Part model, mm, in its own coordinate system. Face numbers are marked on the shaded views. A direction names the side the tool comes from. Give positions to 0.01 mm unless a question says otherwise; leave off trailing zeros. One line per item, written item: value.
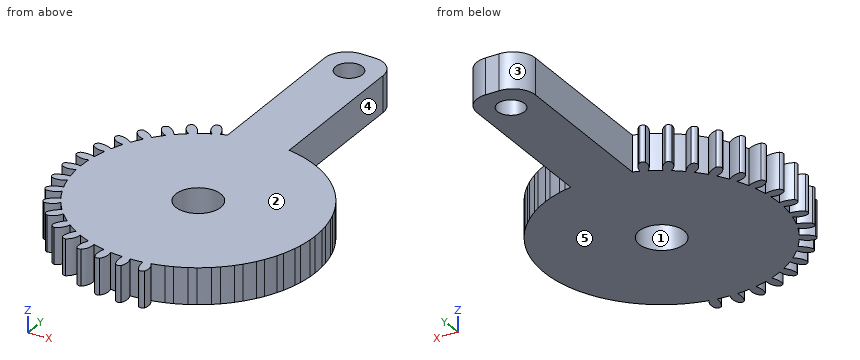
```python
from build123d import *

# Parameters (mm, degrees)
SKETCH1_R           = 13
BOSS_EXTRUDE1_DEPTH = 4
BOSS_EXTRUDE2_DEPTH = 4
CIRPATTERN1_COUNT   = 37
CUT_EXTRUDE1_START  = -6
CUT_EXTRUDE1_DEPTH  = 6
SKETCH5_W           = 6.5
SKETCH5_H           = 20
BOSS_EXTRUDE3_DEPTH = 4
FILLET1_R           = 2.5
SKETCH6_R           = 2.5
CUT_EXTRUDE2_DEPTH  = 36.685455193
SKETCH7_R           = 1.5
CUT_EXTRUDE3_DEPTH  = 36.685455193


with BuildPart() as part:
    # Sketch1 → Boss-Extrude1 (new body)
    with BuildSketch(Plane.XY):
        Circle(SKETCH1_R)
    extrude(amount=BOSS_EXTRUDE1_DEPTH)

    # Sketch2 → Boss-Extrude2 (add)
    with BuildSketch(Plane.XY.offset(4)):
        with BuildLine():
            Line((-1.442756516, 12.919692475), (-0.673396871, 12.982547387))
            ThreePointArc((-0.673396871, 12.982547387), (-0.676161598, 13.791154594), (-0.946073249, 14.553388784))
            ThreePointArc((-0.946073249, 14.553388784), (-1.263795502, 14.68499365), (-1.581517754, 14.553388784))
            ThreePointArc((-1.581517754, 14.553388784), (-1.735779337, 13.717545135), (-1.442756516, 12.919692475))
        make_face()
    boss_extrude2 = extrude(amount=-BOSS_EXTRUDE2_DEPTH)

    # CirPattern1: Boss-Extrude2 ×37 about axis
    cirpattern1_axis = Axis((-0.003550518, 0.04085181, 0), (0, 0, 1))
    for i in range(1, CIRPATTERN1_COUNT):
        add(boss_extrude2.rotate(cirpattern1_axis, i * 360 / CIRPATTERN1_COUNT))

    # Sketch3 → Cut-Extrude1 (cut)
    with BuildSketch(Plane.XY.offset(4).offset(CUT_EXTRUDE1_START)):
        with BuildLine():
            ThreePointArc((2.580226265, -12.741366976), (12.998773331, -0.178582984), (2.929279614, 12.665674911))
            ThreePointArc((2.929279614, 12.665674911), (2.706489738, 14.000196281), (3.492602617, 15.101381624))
            ThreePointArc((3.492602617, 15.101381624), (15.498537433, -0.212925866), (3.076423624, -15.191629856))
            ThreePointArc((3.076423624, -15.191629856), (3.335791003, -13.863732578), (2.580226265, -12.741366976))
        make_face()
    extrude(amount=CUT_EXTRUDE1_DEPTH, mode=Mode.SUBTRACT)

    # Sketch5 → Boss-Extrude3 (add)
    with BuildSketch(Plane.XY.offset(4)):
        with Locations((-1.029483868, 22.275423326)):
            Rectangle(SKETCH5_W, SKETCH5_H)
    extrude(amount=-BOSS_EXTRUDE3_DEPTH)

    # Fillet1
    fillet1_edges = [part.edges().sort_by_distance(p)[0] for p in [
        (2.220516132, 32.275423326, 2),
        (-4.279483868, 32.275423326, 2),
    ]]
    fillet(fillet1_edges, radius=FILLET1_R)

    # Sketch6 → Cut-Extrude2 (cut, through all)
    with BuildSketch(Plane.XY.offset(4)):
        Circle(SKETCH6_R)
    extrude(amount=-CUT_EXTRUDE2_DEPTH, mode=Mode.SUBTRACT)

    # Sketch7 → Cut-Extrude3 (cut, through all)
    with BuildSketch(Plane.XY.offset(4)):
        with Locations((-1.029483868, 28.906928641)):
            Circle(SKETCH7_R)
    extrude(amount=-CUT_EXTRUDE3_DEPTH, mode=Mode.SUBTRACT)


solid = part.part
```
1) Wall check: line 1 along Y through (x, z) = (-10.75, 0.65); line 2 along X through (y, z) = (18.5, 3.8); line 3 along Y through (x, z) = (0, 1.25). Give the ranges that are in metal, low to high. Write a range as [from, to].
Answer:
line 1: y = [-9.85, -8.78], [-7.31, 7.31], [7.49, 8.61]
line 2: x = [-4.28, 2.22]
line 3: y = [-14.66, -2.5], [2.5, 27.82], [30, 32.26]
2) Drop flat-ended pins along their axis: P1, Ø2, axis at y = -9.5, z = 2, coming from the -X side; P2, Ø4, axis at x = 0, y = 0, coming from the -Z side; P3, Ø1.2, axis at y = 18, z = 2, coming from the +X side; P4, Ø2, axis at y = 25, z = 1.5, coming from the -X side. Give the stop position or say it passes through.
Answer:
P1: stops at x = -11.12
P2: passes through
P3: stops at x = 2.22
P4: stops at x = -4.28
3) Two-plate mould, pull along Y, no slides. Class the marked faces 1, 2 and 3: pulls with the +Y half, pulls with the -Y half, needs draft (parallel to the pull), parting line crosses it, or undercut.
Answer:
face 1: undercut
face 2: needs draft
face 3: pulls with the +Y half
4) Which spindle directions (+Z, -Z, +X, -X, +Y, -Y) get a long thin tool onto all of the face, cutting with end or side? Do the marked faces 4 and 5. Say none if no direction does.
Answer:
face 4: +Z, -Z, +X, +Y
face 5: -Z, +X, -X, +Y, -Y
5) Slice it at A-A on z = 2.25. Count the separate pieces of the cut face and the enclosed holes in it, then the cut area to 3 significant figures.
Answer:
separate pieces: 1
enclosed holes: 2
area: 656 mm2
